from build123d import *

# Parameters (mm, degrees)
SKETCH1_W                 = 41.8
SKETCH1_H                 = 143.8
BOSS_EXTRUDE1_DEPTH       = 12
SHELL1_T                  = -7
SHELL1_THICKNESS_2_FACE_W = 27.8
SHELL1_THICKNESS_2_FACE_H = 129.8
SHELL1_THICKNESS_2_DEPTH  = 4
SKETCH2_R                 = 2.2
CUT_EXTRUDE1_DEPTH        = 5.2
SKETCH3_R                 = 2.2
CUT_EXTRUDE2_DEPTH        = 5.2
SKETCH5_R                 = 1.7
CUT_EXTRUDE3_DEPTH        = 10
CHAMFER1_SIZE             = 2
CUT_EXTRUDE4_DEPTH        = 3.5


with BuildPart() as part:
    # Sketch1 → Boss-Extrude1 (new body)
    with BuildSketch(Plane.XY):
        with Locations((0, 71.9)):
            Rectangle(SKETCH1_W, SKETCH1_H)
    extrude(amount=-BOSS_EXTRUDE1_DEPTH)

    # Shell1
    shell1_openings = [part.faces().sort_by_distance(p)[0] for p in [
        (0, 71.9, -12),
    ]]
    offset(amount=SHELL1_T, openings=shell1_openings, kind=Kind.INTERSECTION)

    # Shell1 thickness 2 face (on inner face of the shell) → Shell1 thickness 2 (cut)
    with BuildSketch(Plane(origin=(0, 71.9, -7), x_dir=(1, 0, 0), z_dir=(0, 0, 1))):
        Rectangle(SHELL1_THICKNESS_2_FACE_W, SHELL1_THICKNESS_2_FACE_H)
    extrude(amount=SHELL1_THICKNESS_2_DEPTH, mode=Mode.SUBTRACT)

    # Sketch2 → Cut-Extrude1 (cut)
    with BuildSketch(Plane(origin=(0, 143.8, 0), x_dir=(1, 0, 0), z_dir=(0, 1, 0))):
        with Locations(Location((-15, 6, 0), (0, 0, 270))):
            Circle(SKETCH2_R)
        with Locations(Location((15, 6, 0), (0, 0, 270))):
            Circle(SKETCH2_R)
    cut_extrude1 = extrude(amount=-CUT_EXTRUDE1_DEPTH, mode=Mode.SUBTRACT)

    # Mirror1: Cut-Extrude1 across plane
    add(cut_extrude1.mirror(Plane.ZX.offset(71.9)), mode=Mode.SUBTRACT)

    # Sketch3 → Cut-Extrude2 (cut)
    with BuildSketch(Plane.ZY.offset(20.9)):
        with Locations((-6, 129.4)):
            Circle(SKETCH3_R)
        with Locations((-6, 14.4)):
            Circle(SKETCH3_R)
    extrude(amount=-CUT_EXTRUDE2_DEPTH, mode=Mode.SUBTRACT)

    # Sketch5 → Cut-Extrude3 (cut)
    with BuildSketch(Plane(origin=(0, 0, -3), x_dir=(-1, 0, 0), z_dir=(0, 0, -1))):
        with Locations((-5.75, 63.9)):
            Circle(SKETCH5_R)
        with Locations((-5.75, 79.9)):
            Circle(SKETCH5_R)
    extrude(amount=-CUT_EXTRUDE3_DEPTH, mode=Mode.SUBTRACT)

    # Chamfer1
    chamfer1_edges = [part.edges().sort_by_distance(p)[0] for p in [
        (7.45, 63.9, 0),
        (7.45, 79.9, 0),
    ]]
    chamfer(chamfer1_edges, length=CHAMFER1_SIZE)

    # Sketch6 → Cut-Extrude4 (cut)
    with BuildSketch(Plane(origin=(0, 0, -3), x_dir=(-1, 0, 0), z_dir=(0, 0, -1))):
        with BuildLine():
            Line((11.409552025, 37.4), (11.409552025, 29.4))
            ThreePointArc((11.409552025, 29.4), (9.709552025, 27.7), (8.009552025, 29.4))
            Line((8.009552025, 29.4), (8.009552025, 37.4))
            ThreePointArc((8.009552025, 37.4), (9.709552025, 39.1), (11.409552025, 37.4))
        make_face()
        with BuildLine():
            Line((11.409552025, 106.4), (11.409552025, 114.4))
            ThreePointArc((11.409552025, 114.4), (9.709552025, 116.1), (8.009552025, 114.4))
            Line((8.009552025, 114.4), (8.009552025, 106.4))
            ThreePointArc((8.009552025, 106.4), (9.709552025, 104.7), (11.409552025, 106.4))
        make_face()
        with BuildLine():
            Line((-11.409552025, 106.4), (-11.409552025, 114.4))
            ThreePointArc((-11.409552025, 114.4), (-9.709552025, 116.1), (-8.009552025, 114.4))
            Line((-8.009552025, 114.4), (-8.009552025, 106.4))
            ThreePointArc((-8.009552025, 106.4), (-9.709552025, 104.7), (-11.409552025, 106.4))
        make_face()
        with BuildLine():
            Line((-11.409552025, 37.4), (-11.409552025, 29.4))
            ThreePointArc((-11.409552025, 29.4), (-9.709552025, 27.7), (-8.009552025, 29.4))
            Line((-8.009552025, 29.4), (-8.009552025, 37.4))
            ThreePointArc((-8.009552025, 37.4), (-9.709552025, 39.1), (-11.409552025, 37.4))
        make_face()
    extrude(amount=-CUT_EXTRUDE4_DEPTH, mode=Mode.SUBTRACT)


solid = part.part
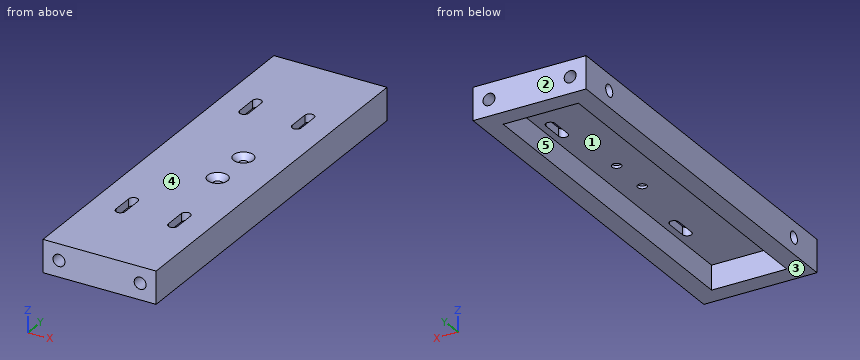
Here's how the part is built. I have some questions about the finished solid (model axes, mm). Face numbers are marked on the shaded views. A direction names the side the tool comes from. Coordinates: 2 decimals unless noted, no trailing zeros. Write each loop counter-clockwise with the first axis right and the second up, starting at its lowest first coordinate (ties: lowest second). Pieces come first, ordered by that corner, then holes.
Item 1: I want a section at B-B on y = 134. Write out the boundary of the cut face in (x, z).
Item 2: If we mould it in two halves opening along Y, with no side actions, what happens to the marked faces 1, 2 and 3? For each: +Y half, -Y half, draft (parallel to the pull), parting line (faces both ways), or undercut.
Item 3: On a 3-axis mill with a long thin cutter (end or side, diameter ignored), from which of +Z, -Z, +X, -X, +Y, -Y can I reach the whole of each face in a straight line? I mean the marked faces 4 and 5. Say none if no direction works.
Item 4: I want a section at D-D on y = 14.4. Write out the boundary of the cut face in (x, z), and give its area (3 significant figures).
Item 5: I want a section at C-C on x = -4.5. Write out the boundary of the cut face in (y, z), and give its area (3 significant figures).
Item 6: If I drill on line 1 (X direction, y = 111, z = -2); line 2 (Y direction, x = -16.75, z = -6); line 3 (X direction, y = 103, z = -7.5), over which ranges is the centre line in solid material (lowest first)?
Item 7: Will these pins go through, and if not, where does the flat tip stop? pin 1 (2 mm diameter, centred on x = 5.75, y = 63.9, fed in from -Z); pin 2 (1.3 mm diameter, centred on x = -15.5, z = -6.5, fed in from +Y).
Findings below:
1. outline: (-20.9, -12) - (-13.9, -12) - (-13.9, -3) - (13.9, -3) - (13.9, -12) - (20.9, -12) - (20.9, 0) - (-20.9, 0) - close
2. face 1: undercut
2. face 2: +Y half
2. face 3: draft
3. face 4: +Z, +X, -X, +Y, -Y
3. face 5: -Z
4. outline: (-20.9, -12) - (-13.9, -12) - (-13.9, -3) - (13.9, -3) - (13.9, -12) - (20.9, -12) - (20.9, 0) - (-20.9, 0) - (-20.9, -3.8) - (-15.7, -3.8) - (-15.7, -8.2) - (-20.9, -8.2) - close
4. area: 229 mm2
5. outline: (0, -12) - (7, -12) - (7, -3) - (136.8, -3) - (136.8, -12) - (143.8, -12) - (143.8, 0) - (0, 0) - close
5. area: 557 mm2
6. line 1: x = -20.9 to -11.41, -8.01 to 8.01, 11.41 to 20.9
6. line 2: y = 5.2 to 12.2, 16.6 to 127.2, 131.6 to 138.6
6. line 3: x = -20.9 to -13.9, 13.9 to 20.9
7. pin 1: passes through
7. pin 2: stops at y = 138.6
